Autodesk Inventor part; units mm, degrees
ref_plane "YZ Plane" through (0, 0, 0) normal (1, 0, 0) x (0, 1, 0)
ref_plane "XZ Plane" through (0, 0, 0) normal (0, 1, 0) x (-1, 0, 0)
ref_plane "XY Plane" through (0, 0, 0) normal (0, 0, 1) x (1, 0, 0)
sketch "Boceto1" plane through (0, 0, 0) normal (0, 0, 1) x (1, 0, 0)
  line L0 (-74, 6) -> (74, 6)
  line L1 (74, 6) -> (74, -6)
  line L2 (74, -6) -> (-74, -6)
  line L3 (-74, -6) -> (-74, 6)
  circle A0 centre (0, 0) radius 1.5
  circle A1 centre (57, 0) radius 1.5
  circle A2 centre (-57, 0) radius 1.5
  circle A3 centre (-9.5, 0) radius 0.65
  circle A4 centre (9.5, 0) radius 0.65
  circle A5 centre (28.5, 0) radius 0.65
  circle A6 centre (47.5, 0) radius 0.65
  circle A7 centre (66.5, 0) radius 0.65
  circle A8 centre (-28.5, 0) radius 0.65
  circle A9 centre (-47.5, 0) radius 0.65
  circle A10 centre (-66.5, 0) radius 0.65
  point P0 (-74, 0)
  point P1 (0, 6)
  dimension "d0" = 148
  dimension "d1" = 12
  dimension "d2" = 3
  dimension "d3" = 3
  dimension "d4" = 3
  dimension "d5" = 57
  dimension "d6" = 57
  dimension "d7" = 1.3
  dimension "d8" = 1.3
  dimension "d9" = 19
  dimension "d10" = 9.5
  dimension "d13" = 19
  dimension "d20" = 19
extrude "Extrusión1" add sketch "Boceto1" along normal blind 12
sketch "Boceto2" plane through (0, 0, 12) normal (0, 0, 1) x (1, 0, 0)
  circle A0 centre (-66.5, 0) radius 0.65
  circle A1 centre (-66.5, 0) radius 2.5
  line L0 (-78, 0) -> (74, 0) construction
  line L1 (74, -6) -> (74, 6) construction
  circle A2 centre (-47.5, 0) radius 2.5
  circle A3 centre (-28.5, 0) radius 2.5
  circle A4 centre (-9.5, 0) radius 2.5
  circle A5 centre (9.5, 0) radius 2.5
  circle A6 centre (28.5, 0) radius 2.5
  circle A7 centre (47.5, 0) radius 2.5
  circle A8 centre (66.5, 0) radius 2.5
  point P0 (0, 0)
  dimension "d27" = 5
  dimension "d30" = 19
  dimension "d35" = 152
extrude "Extrusión2" cut sketch "Boceto2" against normal blind 1.5 contours A0 | A1 | A2 | A3 | A4 | A5 | A6 | A7 | A8
fillet "Empalme1" radius 2 4 edges at (-74, -6, 6) (74, -6, 6) (74, 6, 6) (-74, 6, 6)
equation "\"d8\" = d7"
properties part number "Guia fibra 8Ch V2_2"
Geometry check sheet. Reference: the model listing, model coordinates, mm. A direction names the side the tool comes from. Round coordinates to 2 decimals unless told otherwise and drop trailing zeros. Loops run counter-clockwise (first coordinate to the right, second up) from the corner with the lowest first, then second, coordinate; pieces in that order, holes last. Notation, with made-up numbers: (-23, -12.5) - (27, -12.5) arc R16 ccw to (27, 15.5) - close; hole circle Ø10 at (33, 45.25). An arc over 180 degrees is marked (long way). Use a Markdown table: item, result.
Q1. Cross-section at A-A on x = -57. Record the cut outline in (y, z), plus the area to 3 significant figures.
Solutions:
| item | result |
|---|---|
| outline | (-6, 0) - (-1.5, 0) - (-1.5, 12) - (-6, 12) - close; (1.5, 0) - (6, 0) - (6, 12) - (1.5, 12) - close |
| area | 108 mm2 |
Q2. Draft check along X on faces 3 (the flat face through (-74, 0, 6)), 4 (the cylindrical face through (-1.5, -0.07, 5.92)), 5 (the flat face through (-1, 1.4, 0)). Enter one of: released by +X, released by -X, zero draft, split by the parting line, or undercut.
Solutions:
| item | result |
|---|---|
| face 3 | released by -X |
| face 4 | undercut |
| face 5 | zero draft |
Q3. Access from +Z, -Z, +X, -X, +Y, -Y to the whole of each face (thin tool, end or side, straight path). Record for faces 1 (the flat face through (67, -1, 10.5)), 2 (the cylindrical face through (58.43, -0.45, 5.92)).
Solutions:
| item | result |
|---|---|
| face 1 | +Z |
| face 2 | +Z, -Z |
Q4. Material ranges on line 1 (Y direction, x = 47.5, z = 6); line 2 (Y direction, x = -57, z = 4.5); line 3 (X direction, y = 0.75, z = 2), recorded low to high.
Solutions:
| item | result |
|---|---|
| line 1 | y = -6 to -0.65, 0.65 to 6 |
| line 2 | y = -6 to -1.5, 1.5 to 6 |
| line 3 | x = -74 to -58.3, -55.7 to -1.3, 1.3 to 55.7, 58.3 to 74 |
Q5. Cross-section at B-B on z = 8.75. State how many separate pieces and enclosed holes the cut face has, plus the area to 3 significant figures.
Solutions:
| item | result |
|---|---|
| separate pieces | 1 |
| enclosed holes | 11 |
| area | 1,740 mm2 |
Q6. Go/stop test with flat-tipped pins: P1, Ø4, axis at x = -9.5, y = 0, coming from the +Z side; P2, Ø0.8, axis at x = 47.5, y = 0, coming from the -Z side. Record where each tip stops, or that it passes through.
Solutions:
| item | result |
|---|---|
| P1 | stops at z = 10.5 |
| P2 | passes through |
